from build123d import *

# Parameters (mm, degrees)
F0_W     = 190
F0_H     = 9.6947368307
F0_H_2   = 10.6105263385
F0_W_2   = 5
F1_DEPTH = 10
F2_DEPTH = 13
F3_DEPTH = 30


with BuildPart() as f1:
    # F0 (on Top) → F1 (new body)
    with BuildSketch(Plane.XY):
        Polygon((-95, 15), (-120, 15), (-120, -15), (-95, -15), (-95, -5.3052631693), (-100, -5.3052631693), (-100, 5.3052631693), (-95, 5.3052631693), align=None)
        with Locations((0, 10.1526315846)):
            Rectangle(F0_W, F0_H)
        Polygon((120, 15), (95, 15), (95, 5.3052631693), (100, 5.3052631693), (100, -5.3052631693), (95, -5.3052631693), (95, -15), (120, -15), align=None)
        with Locations((0, -10.1526315846)):
            Rectangle(F0_W, F0_H)
        Rectangle(F0_W, F0_H_2)
        with Locations((-97.5, 0)):
            Rectangle(F0_W_2, F0_H_2)
        with Locations((97.5, 0)):
            Rectangle(F0_W_2, F0_H_2)
    extrude(amount=F1_DEPTH)

    # F0 (on Top) → F2 (join)
    with BuildSketch(Plane.XY):
        Polygon((-95, 15), (-120, 15), (-120, -15), (-95, -15), (-95, -5.3052631693), (-100, -5.3052631693), (-100, 5.3052631693), (-95, 5.3052631693), align=None)
        with Locations((0, 10.1526315846)):
            Rectangle(F0_W, F0_H)
        Polygon((120, 15), (95, 15), (95, 5.3052631693), (100, 5.3052631693), (100, -5.3052631693), (95, -5.3052631693), (95, -15), (120, -15), align=None)
        with Locations((0, -10.1526315846)):
            Rectangle(F0_W, F0_H)
    extrude(amount=F2_DEPTH)

    # F0 (on Top) → F3 (join)
    with BuildSketch(Plane.XY):
        Polygon((-95, 15), (-120, 15), (-120, -15), (-95, -15), (-95, -5.3052631693), (-100, -5.3052631693), (-100, 5.3052631693), (-95, 5.3052631693), align=None)
        Polygon((120, 15), (95, 15), (95, 5.3052631693), (100, 5.3052631693), (100, -5.3052631693), (95, -5.3052631693), (95, -15), (120, -15), align=None)
    extrude(amount=F3_DEPTH)


solid = f1.part
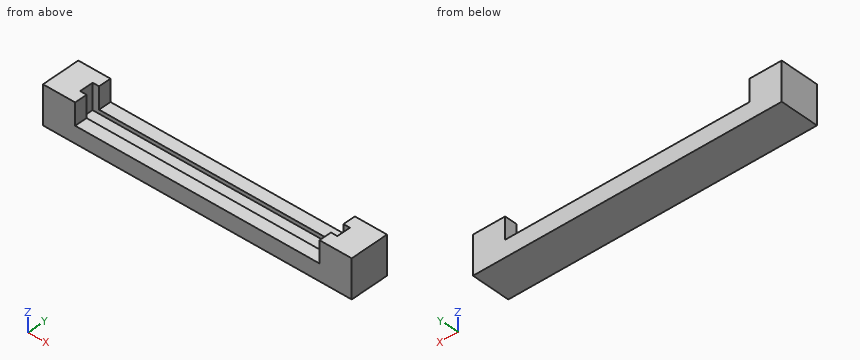
CAD build for the part. Positions are in the model's coordinates, mm. Round coordinates to 2 decimals unless told otherwise and drop trailing zeros. Order: outer loops, then holes, each group sorted by start corner. A loop starts at its lowest first (then second) coordinate and runs counter-clockwise, first axis right, second up. Notation, with made-up numbers: (38.5, 37.25) - (78.5, 37.25) arc R20 cw to (78.5, 73.25) - close; hole circle Ø7 at (75.25, 2.5). An arc over 180 degrees is marked (long way). Return JSON: item names as keys, results as strings.
(1) Wall check: probe 1 along X at (y, z) = (-4, 16); probe 2 along X at (y, z) = (5.5, 16); probe 3 along Y at (x, z) = (21, 12.75). Give the ranges that are in metal, low to high. Write a range as from..to.
Answer key:
{"probe 1": "x = -120..-100, 100..120", "probe 2": "x = -120..-95, 95..120", "probe 3": "y = -15..-5.31, 5.31..15"}
(2) Cut at C-C (x = -83). Give the cut face in (y, z).
Answer key:
{"outline": "(-15, 0) - (15, 0) - (15, 13) - (5.31, 13) - (5.31, 10) - (-5.31, 10) - (-5.31, 13) - (-15, 13) - close"}
(3) Cut at A-A (z = 18). Give the cut face in (x, y).
Answer key:
{"outline": "(-120, -15) - (-95, -15) - (-95, -5.31) - (-100, -5.31) - (-100, 5.31) - (-95, 5.31) - (-95, 15) - (-120, 15) - close; (95, -15) - (120, -15) - (120, 15) - (95, 15) - (95, 5.31) - (100, 5.31) - (100, -5.31) - (95, -5.31) - close"}
(4) Pin check, flat tips, straight feed: pin 1 Ø3 at (x, y) = (-27.5, -8) entering from +Z; pin 2 Ø2 at (x, y) = (58.5, 3) entering from +Z. Stop position of each tip, or through.
Answer key:
{"pin 1": "stops at z = 13", "pin 2": "stops at z = 10"}
(5) Cut at B-B (y = 11.75). Give the cut face in (x, z), then the cut area to 3 significant figures.
Answer key:
{"outline": "(-120, 0) - (120, 0) - (120, 30) - (95, 30) - (95, 13) - (-95, 13) - (-95, 30) - (-120, 30) - close", "area": "3,970 mm^2"}
